Design review of the part built by this model. Coordinates are the model's own, in mm. A direction names the side the tool comes from. Coordinates: 2 decimals unless noted, no trailing zeros. Write each loop counter-clockwise with the first axis right and the second up, starting at its lowest first coordinate (ties: lowest second). Pieces come first, ordered by that corner, then holes. Notation, with made-up numbers: (-11, 53) -> (46, 53) arc R23 cw to (46, 70) -> close; hole circle Ø7 at (-27.5, 40). An arc over 180 degrees is marked (long way). One line per question, with ' | ' between items. Start each with the question number.
Q1. Draft analysis for pull direction X (two halves, no side actions). For faces 1 (the cylindrical face through (2.85, 42.5, -3.01)), 2 (the flat face through (45, 13, -12.828)), 3 (the flat face through (6, 0, -88)), state which applies: pulls with the +X half, pulls with the -X half, needs draft (parallel to the pull), parting line crosses it, or undercut.
Q2. For faces 4 (the flat face through (12.828, 13, -88)), 5 (the cylindrical face through (86.05, 42.5, -174.79)), list the 3-axis set-ups (+Z, -Z, +X, -X, +Y, -Y) from which the entire face can be reached by the end or side of a thin tool; tool diameter is ignored.
Q3. Wall thickness on probe 1 along X at (y, z) = (21.5, -27.5); probe 2 along Z at (x, y) = (23, 17); probe 3 along Y at (x, z) = (46, -67.5): over which ranges is each line inside the solid? List them lowest first.
Q4. Add section C-C on x = 72. State the section outline as (y, z) points, and give its area (3 significant figures).
Q5. Add section A-A on y = 20. State the section outline as (x, z) points.
Q6. Add section B-B on z = -63. State the section outline as (x, y) points, and give its area (3 significant figures).
Q7. For P1, Ø7.5, axis at y = 9, z = -88.5, coming from the -X side; P2, Ø1, axis at x = 9, y = 36.5, coming from the +Z side; P3, Ø2, axis at x = 30, z = -143, coming from the -Y side, all flat-tipped, find the tip position at first contact; note any pin that passes through.
Autodesk Inventor part; units mm, degrees
ref_plane "YZ Plane" through (0, 0, 0) normal (1, 0, 0) x (0, 1, 0)
ref_plane "XZ Plane" through (0, 0, 0) normal (0, 1, 0) x (-1, 0, 0)
ref_plane "XY Plane" through (0, 0, 0) normal (0, 0, 1) x (1, 0, 0)
sketch "Sketch1" plane through (0, 0, 0) normal (0, 1, 0) x (-1, 0, 0)
  line L0 (0, 0) -> (-88.9, 0)
  line L1 (-88.9, 0) -> (-88.9, -177.8)
  line L2 (-88.9, -177.8) -> (0, -177.8)
  line L3 (0, -177.8) -> (0, 0)
  dimension "d0" = 177.8
  dimension "d1" = 88.9
extrude "Extrusion1" add sketch "Sketch1" along normal blind 83.82
sketch "Sketch2" plane through (0, 0, 0) normal (0, -1, 0) x (1, 0, 0)
  point P0 (0, 0)
sketch "Sketch3" plane through (0, 0, 0) normal (0, -1, 0) x (1, 0, 0)
  line L0 (88.9, 0) -> (88.9, -177.8)
  line L1 (0, 0) -> (88.9, 0)
  line L2 (0, -177.8) -> (0, 0)
  line L3 (88.9, -177.8) -> (0, -177.8)
  line L4 (76.0718, -164.9718) -> (76.0718, -12.8282)
  line L5 (76.0718, -12.8282) -> (12.8282, -12.8282)
  line L6 (12.8282, -12.8282) -> (12.8282, -164.9718)
  line L7 (12.8282, -164.9718) -> (76.0718, -164.9718)
extrude "Extrusion2" cut sketch "Sketch3" against normal blind 25.4 contours L7 L6 L5 L4
fillet "Fillet1" radius 10 4 edges at (88.9, 41.91, -177.8) (0, 41.91, -177.8) (88.9, 41.91, 0) (0, 41.91, 0)
properties part number "Capstone"
Output values:
1) face 1: pulls with the -X half | face 2: undercut | face 3: needs draft
2) face 4: -Y | face 5: -Z, +X, +Y, -Y
3) probe 1: x = 0 to 12.83, 76.07 to 88.9 | probe 2: z = -177.8 to -164.97, -12.83 to 0 | probe 3: y = 25.4 to 83.82
4) outline: (0, -177.8) -> (83.82, -177.8) -> (83.82, 0) -> (0, 0) -> (0, -12.83) -> (25.4, -12.83) -> (25.4, -164.97) -> (0, -164.97) -> close | area: 11,000 mm2
5) outline: (0, -167.8) arc R10 ccw to (10, -177.8) -> (78.9, -177.8) arc R10 ccw to (88.9, -167.8) -> (88.9, -10) arc R10 ccw to (78.9, 0) -> (10, 0) arc R10 ccw to (0, -10) -> close; hole (12.83, -164.97) -> (76.07, -164.97) -> (76.07, -12.83) -> (12.83, -12.83) -> close
6) outline: (0, 0) -> (12.83, 0) -> (12.83, 25.4) -> (76.07, 25.4) -> (76.07, 0) -> (88.9, 0) -> (88.9, 83.82) -> (0, 83.82) -> close | area: 5,850 mm2
7) P1: stops at x = 0 | P2: stops at z = -0.01 | P3: stops at y = 25.4
